from build123d import *

# Parameters (mm, degrees)
SKETCH1_R           = 2
BOSS_EXTRUDE1_DEPTH = 1.25
FILLET1_R           = 20


with BuildPart() as part:
    # Sketch1 → Boss-Extrude1 (new, symmetric)
    with BuildSketch(Plane(origin=(0, 0, 0), x_dir=(1, 0, 0), z_dir=(0, 1, 0))):
        Polygon((30, -12.5), (30, 12.5), (-30, 12.5), (-30, -12.5), (-24.69, -12.5), (-24.69, -17.5), (-19.69, -17.5), (-19.69, -12.5), (19.69, -12.5), (19.69, -17.5), (24.69, -17.5), (24.69, -12.5), align=None)
        with Locations(Location((0, 0, 0), (0, 0, 270))):
            Circle(SKETCH1_R, mode=Mode.SUBTRACT)
    extrude(amount=BOSS_EXTRUDE1_DEPTH, both=True)

    # Fillet1
    fillet1_edges = [part.edges().sort_by_distance(p)[0] for p in [
        (-30, 0, -12.5),
        (30, 0, -12.5),
    ]]
    fillet(fillet1_edges, radius=FILLET1_R)


solid = part.part
Check sheet for the modelled part. Datum: model origin and axes. Units: mm. A direction names the side the tool comes from. Give positions to 0.01 mm unless a question says otherwise; leave off trailing zeros. Write each loop counter-clockwise with the first axis right and the second up, starting at its lowest first coordinate (ties: lowest second). Pieces come first, ordered by that corner, then holes. Notation, with made-up numbers: (24, 61.25) -> (53, 61.25) arc R21 ccw to (53, 100.25) -> close; hole circle Ø1 at (-13.5, -12). An arc over 180 degrees is marked (long way). Write item = value, one per line.
Item 1: Scan lines: probe 1 along X at (y, z) = (-0.65, 16); probe 2 along Z at (x, y) = (-7, -1.1); probe 3 along X at (y, z) = (-0.95, -1). Record each from-to range of solid material in increasing order. Write a range as from..to.
Output:
probe_1 = -24.69..-19.69, 19.69..24.69
probe_2 = -12.5..12.5
probe_3 = -28.1..-1.73, 1.73..28.1
Item 2: Release check for a two-part mould opening along X. For faces 4 (the flat face through (-27, 0, 12.5)), 5 (the cylindrical face through (24.297, 0.018, -6.486)), 6 (the cylindrical face through (-2, 0, 0)) record: +X half, -X half, draft (parallel to the pull), parting line (faces both ways), or undercut.
Output:
face_4 = draft
face_5 = +X half
face_6 = undercut
Item 3: Sectioned sample at B-B on z = 0. Record the boundary of the cut face in (x, y).
Output:
outline = (-28.54, -1.25) -> (-2, -1.25) -> (-2, 1.25) -> (-28.54, 1.25) -> close; (2, -1.25) -> (28.54, -1.25) -> (28.54, 1.25) -> (2, 1.25) -> close
Item 4: Sectioned sample at C-C on y = 0.65. Record the boundary of the cut face in (x, z), and give its area (3 significant figures).
Output:
outline = (-30, 7.5) arc R20 ccw to (-10, -12.5) -> (10, -12.5) arc R20 ccw to (30, 7.5) -> (30, 12.5) -> (24.69, 12.5) -> (24.69, 17.5) -> (19.69, 17.5) -> (19.69, 12.5) -> (-19.69, 12.5) -> (-19.69, 17.5) -> (-24.69, 17.5) -> (-24.69, 12.5) -> (-30, 12.5) -> close; hole circle Ø4 at (0, 0)
area = 1,370 mm^2
Item 5: Tool access check on faces 1 (the flat face through (-24.69, 0, 15)), 2 (the flat face through (-19.69, 0, 15)), 3 (the flat face through (27, 0, 12.5)). Record the directions out of +Z, -Z, +X, -X, +Y, -Y that give a thin tool (end or side, any length) a straight path to the whole face; none if there is none.
Output:
face_1 = +Z, -X, +Y, -Y
face_2 = +Z, +Y, -Y
face_3 = +Z, +X, +Y, -Y
Item 6: Sectioned sample at D-D on z = -8.5. Record the boundary of the cut face in (x, y).
Output:
outline = (-22, -1.25) -> (22, -1.25) -> (22, 1.25) -> (-22, 1.25) -> close
Item 7: Sectioned sample at A-A on x = 0. Record the boundary of the cut face in (y, z), and give its area (3 significant figures).
Output:
outline = (-1.25, -12.5) -> (1.25, -12.5) -> (1.25, -2) -> (-1.25, -2) -> close; (-1.25, 2) -> (1.25, 2) -> (1.25, 12.5) -> (-1.25, 12.5) -> close
area = 52.5 mm^2
Item 8: Gauge pin test, flat end, axial feed: pin 1 (1.2 mm diameter, centred on x = 6.5, y = 0, fed in from +Z). Record the tip position at first contact, or that the pin passes through.
Output:
pin_1 = 12.5
